Verification items for the finished model (mm, model axes). Face numbers are marked on the shaded views. A direction names the side the tool comes from. Round coordinates to 2 decimals unless told otherwise and drop trailing zeros.
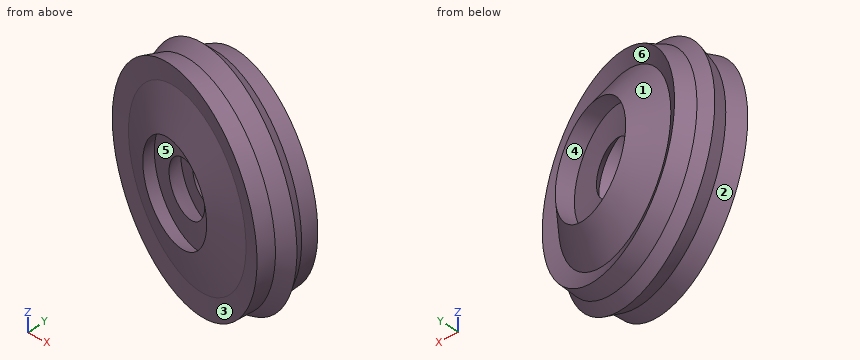
from build123d import *


with BuildPart() as f1:
    # F0 (on Top) → F1 (revolve)
    with BuildSketch(Plane.XY):
        Polygon((-115.35806, -15.976095), (-127.390557, -22.441317), (-124.337537, -38.245195), (-132.059885, -54.228663), (-112.484628, -58.000044), (-78.36262, -80.089555), (-80.697283, -64.465263), (-55.554753, -76.138583), (-63.456689, -54.228663), (-43.70184, -62.66937), (-52.86091, -31.959562), (-39.032516, -26.931056), (-64.175046, -15.976095), (-58.248594, 0.18696), (-93.807319, -10.767997), (-106.019405, -1.249754), align=None)
    revolve(axis=Axis((-21.009779, -52.6792, 0), (-0.29869, -0.95435, 0)))


solid = f1.part
Q1. Release check for a two-part mould opening along Y. For the marked faces 1, 2, 3 and 4 record: released by +Y, released by -Y, zero draft, split by the parting line, or undercut.
Recorded:
face 1: released by +Y
face 2: undercut
face 3: released by -Y
face 4: undercut
Q2. Tool access check on the marked faces 5 and 6. Record the directions out of +Z, -Z, +X, -X, +Y, -Y that give a thin tool (end or side, any length) a straight path to the whole face; none if there is none.
Recorded:
face 5: none
face 6: +Y
Q3. Depth check by flat-ended pin: P1, Ø1.5, axis at y = -15, z = 27.5, coming from the -X side; P2, Ø1, axis at x = -99.5, z = 1.5, coming from the -Y side; P3, Ø3, axis at y = -19, z = -73.5, coming from the +X side. Enter the tip coordinate at first touch or a pass-through.
Recorded:
P1: stops at x = -110.89
P2: stops at y = -66.72
P3: stops at x = -57.53
Q4. Sectioned sample at A-A (z = 33). Give the number of separate pieces and of enclosed holes in the cut face, plus the area to 3 significant figures.
Recorded:
separate pieces: 1
enclosed holes: 2
area: 11,000 mm2
Q5. Material ranges on line 1 along Y through (x, z) = (15.5, 7.5); line 2 along Y through (x, z) = (-35, -27); line 3 along Y through (x, z) = (-88, 84.5), recorded low to high.
Recorded:
line 1: y = -107.91 to -101.82, -95.3 to -54.15, -52.57 to -43.1
line 2: y = -82.38 to -80.49, -64.33 to -46.19, -34.58 to -27.14
line 3: y = -67.76 to -60.85, -38.72 to -33.63
